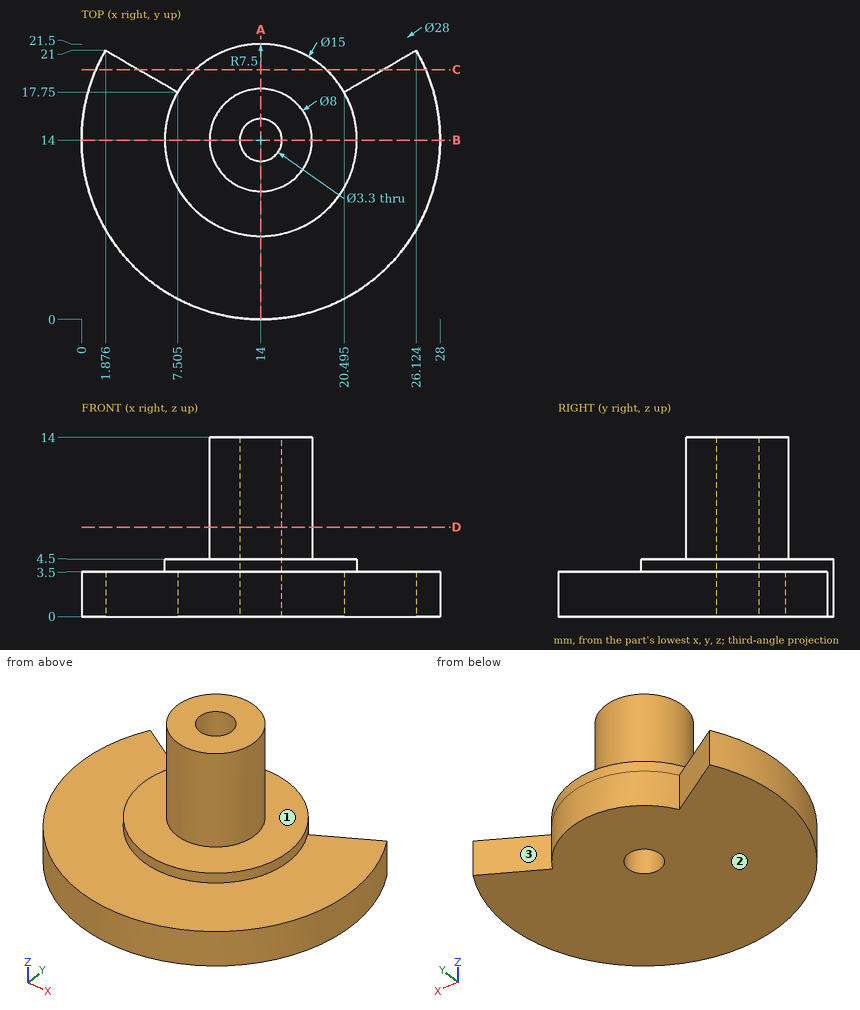
Input: dimensioned drawing with shaded views. Units: mm. Origin: part minimum x, y, z. A direction names the side the tool comes from. Give positions to 0.01 mm unless a question says otherwise; leave off trailing zeros. Order: outer loops, then holes, each group sorted by start corner. A loop starts at its lowest first (then second) coordinate and runs counter-clockwise, first axis right, second up. Notation, with made-up numbers: (1.5, -2) -> (42.5, -2) arc R16 ccw to (42.5, 12) -> close; hole circle Ø8 at (-18, 23.25). An arc over 180 degrees is marked (long way). Use a Markdown table: item, result.
1) Section query A-A, the plane x = 14. Return the cut outline in (y, z).
Answer list:
| item | result |
|---|---|
| outline | (0, 0) -> (12.35, 0) -> (12.35, 14) -> (10, 14) -> (10, 4.5) -> (6.5, 4.5) -> (6.5, 3.5) -> (0, 3.5) -> close; (15.65, 0) -> (21.5, 0) -> (21.5, 4.5) -> (18, 4.5) -> (18, 14) -> (15.65, 14) -> close |
2) Contact query for flat-ended pins moving along their axis: P1, Ø6, axis at x = 9, z = 10, coming from the -Y side (1 decimal); P2, Ø4, axis at x = 22.5, z = 4.5, coming from the +Y side; P3, Ø4, axis at y = 17, z = 4.5, coming from the +X side. Output: stop coordinate, or through.
Answer list:
| item | result |
|---|---|
| P1 | y = 10.5 |
| P2 | y = 19.91 |
| P3 | x = 27.94 |
3) Section query B-B, the plane y = 14. Return the cut outline in (x, z), then the cut area to 3 significant figures.
Answer list:
| item | result |
|---|---|
| outline | (0, 0) -> (12.35, 0) -> (12.35, 14) -> (10, 14) -> (10, 4.5) -> (6.5, 4.5) -> (6.5, 3.5) -> (0, 3.5) -> close; (15.65, 0) -> (28, 0) -> (28, 3.5) -> (21.5, 3.5) -> (21.5, 4.5) -> (18, 4.5) -> (18, 14) -> (15.65, 14) -> close |
| area | 143 mm² |
4) Reachability of the marked faces 1, 2 and 3 from +Z, -Z, +X, -X, +Y, -Y: full face, straight path, thin tool, end or side. Return the list, or none.
Answer list:
| item | result |
|---|---|
| face 1 | +Z |
| face 2 | -Z, +X, -X, +Y, -Y |
| face 3 | +Z, -Z, +Y |
5) Section query D-D, the plane z = 7. Return the cut outline in (x, y), then the cut area to 3 significant figures.
Answer list:
| item | result |
|---|---|
| outline | circle Ø8 at (14, 14); hole circle Ø3.3 at (14, 14) |
| area | 41.7 mm² |
6) Section query C-C, the plane y = 19.5. Return the cut outline in (x, z) (1 decimal).
Answer list:
| item | result |
|---|---|
| outline | (1.1, 0) -> (4.5, 0) -> (4.5, 3.5) -> (1.1, 3.5) -> close; (8.9, 0) -> (19.1, 0) -> (19.1, 4.5) -> (8.9, 4.5) -> close; (23.5, 0) -> (26.9, 0) -> (26.9, 3.5) -> (23.5, 3.5) -> close |
7) Ray query, line 1 along Y through (x, z) = (14, 5.5); line 2 along Y through (x, z) = (14, 3); line 3 along Z through (x, y) = (19.5, 1.5). Return the intervals inside material, ascending. Write a range as [from, to].
Answer list:
| item | result |
|---|---|
| line 1 | [10, 12.35], [15.65, 18] |
| line 2 | [0, 12.35], [15.65, 21.5] |
| line 3 | [0, 3.5] |
